Geometry: final body of the model. Coordinates: model frame, mm. A direction names the side the tool comes from. Give positions to 0.01 mm unless a question says otherwise; leave off trailing zeros. Loops run counter-clockwise (first coordinate to the right, second up) from the corner with the lowest first, then second, coordinate; pieces in that order, holes last.
from build123d import *

# Parameters (mm, degrees)
F0_R     = 30.75
F1_DEPTH = 5.5
F2_DEPTH = 2


with BuildPart() as f1:
    # F0 (on Top) → F1 (new body)
    with BuildSketch(Plane.XY):
        Circle(F0_R)
        with BuildLine():
            ThreePointArc((0, -30), (-21.213203, -21.213203), (-30, 0))
            ThreePointArc((-30, 0), (-21.213203, 21.213203), (0, 30))
            ThreePointArc((0, 30), (21.213203, 21.213203), (30, 0))
            ThreePointArc((30, 0), (21.213203, -21.213203), (0, -30))
        make_face(mode=Mode.SUBTRACT)
    extrude(amount=F1_DEPTH)

    # F0 (on Top) → F2 (join)
    with BuildSketch(Plane.XY):
        with BuildLine():
            Line((-30, 0), (0, 0))
            Line((0, 0), (0, 30))
            ThreePointArc((0, 30), (-21.213203, 21.213203), (-30, 0))
        make_face()
        with BuildLine():
            Line((-5, 24.494897), (-5, 5))
            Line((-5, 5), (-24.494897, 5))
            ThreePointArc((-24.494897, 5), (-17.67767, 17.67767), (-5, 24.494897))
        make_face(mode=Mode.SUBTRACT)
        with BuildLine():
            Line((0, 30), (0, 0))
            Line((0, 0), (30, 0))
            ThreePointArc((30, 0), (21.213203, 21.213203), (0, 30))
        make_face()
        with BuildLine():
            Line((24.494897, 5), (5, 5))
            Line((5, 5), (5, 24.494897))
            ThreePointArc((5, 24.494897), (17.67767, 17.67767), (24.494897, 5))
        make_face(mode=Mode.SUBTRACT)
        with BuildLine():
            Line((30, 0), (0, 0))
            Line((0, 0), (0, -30))
            ThreePointArc((0, -30), (21.213203, -21.213203), (30, 0))
        make_face()
        with BuildLine():
            Line((5, -24.494897), (5, -5))
            Line((5, -5), (24.494897, -5))
            ThreePointArc((24.494897, -5), (17.67767, -17.67767), (5, -24.494897))
        make_face(mode=Mode.SUBTRACT)
        with BuildLine():
            Line((0, -30), (0, 0))
            Line((0, 0), (-30, 0))
            ThreePointArc((-30, 0), (-21.213203, -21.213203), (0, -30))
        make_face()
        with BuildLine():
            Line((-24.494897, -5), (-5, -5))
            Line((-5, -5), (-5, -24.494897))
            ThreePointArc((-5, -24.494897), (-17.67767, -17.67767), (-24.494897, -5))
        make_face(mode=Mode.SUBTRACT)
    extrude(amount=F2_DEPTH)


solid = f1.part
Item 1: Set-up query: faces 1 (the face through (15, -5, 1)), 2 (the face through (0, 0, 2)), 3 (the face through (0, 0, 0)). Return all of +Z, -Z, +X, -X, +Y, -Y with unobstructed straight access to the full face (end or side cutting, diameter ignored); none if empty.
Values follow:
face 1: +Z, -Z
face 2: +Z
face 3: -Z, +X, -X, +Y, -Y
Item 2: Section query D-D on x = -2. Return loops of the section in (y, z).
Values follow:
outline: (-30.68, 0) - (30.68, 0) - (30.68, 5.5) - (29.93, 5.5) - (29.93, 2) - (-29.93, 2) - (-29.93, 5.5) - (-30.68, 5.5) - close
Item 3: Section query A-A on y = 18. Return loops of the section in (x, z), plus the area to 3 significant figures.
Values follow:
outline: (-24.93, 0) - (-17.35, 0) - (-17.35, 2) - (-24, 2) - (-24, 5.5) - (-24.93, 5.5) - close; (-5, 0) - (5, 0) - (5, 2) - (-5, 2) - close; (17.35, 0) - (24.93, 0) - (24.93, 5.5) - (24, 5.5) - (24, 2) - (17.35, 2) - close
area: 56.8 mm2
Item 4: Draft query along Y for faces 4 (the face through (6.7, -29.5, 5.5)), 5 (the face through (-17.822, 17.533, 0.986)), 6 (the face through (14.19, -27.28, 2.71)). Return one class per face: +Y half, -Y half, draft (parallel to the pull), parting line (faces both ways), or undercut.
Values follow:
face 4: draft
face 5: undercut
face 6: parting line
Item 5: Ray query, probe 1 along Y at (x, z) = (8, 0.6); probe 2 along Y at (x, z) = (8.5, 1.6); probe 3 along X at (y, z) = (-19, 0.9). Return the intervals inside material, ascending.
Values follow:
probe 1: y = -29.69 to -23.69, -5 to 5, 23.69 to 29.69
probe 2: y = -29.55 to -23.51, -5 to 5, 23.51 to 29.55
probe 3: x = -24.18 to -16.25, -5 to 5, 16.25 to 24.18
Item 6: Pin query (flat end, axial travel): pin 1 (3 mm diameter, centred on y = 9.5, z = 4, fed in from +X); pin 2 (1 mm diameter, centred on x = -20, z = 4, fed in from -Y); pin 3 (1 mm diameter, centred on y = 10.5, z = 1, fed in from +X). Return the tip coordinate at first contact, or that it passes through.
Values follow:
pin 1: stops at x = 29.69
pin 2: stops at y = -23.78
pin 3: stops at x = 29.08
Item 7: Section query B-B on z = 3.2. Return loops of the section in (x, y).
Values follow:
outline: circle Ø61.5 at (0, 0); hole (-30, 0) arc R30 ccw to (0, -30) arc R30 ccw to (30, 0) arc R30 ccw to (0, 30) arc R30 ccw to start
Item 8: Section query C-C on x = 7.5. Return loops of the section in (y, z), plus the area to 3 significant figures.
Values follow:
outline: (-29.82, 0) - (-23.85, 0) - (-23.85, 2) - (-29.05, 2) - (-29.05, 5.5) - (-29.82, 5.5) - close; (-5, 0) - (5, 0) - (5, 2) - (-5, 2) - close; (23.85, 0) - (29.82, 0) - (29.82, 5.5) - (29.05, 5.5) - (29.05, 2) - (23.85, 2) - close
area: 49.3 mm2
